```python
from build123d import *

# Parameters (mm, degrees)
SKETCH1_W           = 86.9
SKETCH1_H           = 86.9
BOSS_EXTRUDE1_DEPTH = 2
SKETCH2_R           = 1.65
CUT_EXTRUDE3_DEPTH  = 123.911431527
SKETCH3_R           = 1.5
CUT_EXTRUDE4_DEPTH  = 10
SKETCH4_R           = 1.5
CUT_EXTRUDE5_DEPTH  = 10
SKETCH5_W           = 3.5
SKETCH5_H           = 75
SKETCH5_W_2         = 75
SKETCH5_H_2         = 3.5
CUT_EXTRUDE6_DEPTH  = 123.911431527


with BuildPart() as part:
    # Sketch1 → Boss-Extrude1 (new body)
    with BuildSketch(Plane(origin=(0, 0, 0), x_dir=(0, 1, 0), z_dir=(0, 0, 1))):
        with Locations((43.45, 43.45)):
            Rectangle(SKETCH1_W, SKETCH1_H)
    extrude(amount=BOSS_EXTRUDE1_DEPTH)

    # Sketch2 → Cut-Extrude3 (cut, through all)
    with BuildSketch(Plane.XY.offset(2)):
        with Locations((-84.05, 2.85)):
            Circle(SKETCH2_R)
        with Locations((-2.85, 2.85)):
            Circle(SKETCH2_R)
        with Locations((-2.85, 84.05)):
            Circle(SKETCH2_R)
        with Locations((-84.05, 84.05)):
            Circle(SKETCH2_R)
    extrude(amount=-CUT_EXTRUDE3_DEPTH, mode=Mode.SUBTRACT)

    # Sketch3 → Cut-Extrude4 (cut)
    with BuildSketch(Plane.XY.offset(2)):
        with Locations((-79.2, 62.2)):
            Circle(SKETCH3_R)
        with Locations((-41.7, 62.2)):
            Circle(SKETCH3_R)
        with Locations((-41.7, 24.7)):
            Circle(SKETCH3_R)
        with Locations((-79.2, 24.7)):
            Circle(SKETCH3_R)
    extrude(amount=-CUT_EXTRUDE4_DEPTH, mode=Mode.SUBTRACT)

    # Sketch4 → Cut-Extrude5 (cut)
    with BuildSketch(Plane.XY.offset(2)):
        with Locations((-31.5, 66.7)):
            Circle(SKETCH4_R)
        with Locations((-8.5, 66.7)):
            Circle(SKETCH4_R)
        with Locations((-8.5, 20.2)):
            Circle(SKETCH4_R)
        with Locations((-31.5, 20.2)):
            Circle(SKETCH4_R)
    extrude(amount=-CUT_EXTRUDE5_DEPTH, mode=Mode.SUBTRACT)

    # Sketch5 → Cut-Extrude6 (cut, through all)
    with BuildSketch(Plane.XY.offset(2)):
        with Locations((-1.75, 43.45)):
            Rectangle(SKETCH5_W, SKETCH5_H)
        with Locations((-43.45, 85.15)):
            Rectangle(SKETCH5_W_2, SKETCH5_H_2)
    extrude(amount=-CUT_EXTRUDE6_DEPTH, mode=Mode.SUBTRACT)


solid = part.part
```
Here's how the part is built. I have some questions about the finished solid (model axes, mm). A direction names the side the tool comes from. Coordinates: 2 decimals unless noted, no trailing zeros. Order: outer loops, then holes, each group sorted by start corner. A loop starts at its lowest first (then second) coordinate and runs counter-clockwise, first axis right, second up.
Item 1: I'm going to push flat-ended pins straight in: pin 1 Ø6 at (x, y) = (-11, 16.5) entering from -Z; pin 2 Ø0.6 at (x, z) = (-39, 1.5) entering from +Y; pin 3 Ø1 at (y, z) = (29.5, 1.5) entering from +X. Where does each tip first touch, or does it pass through?
Response values:
pin 1: stops at z = 0
pin 2: stops at y = 83.4
pin 3: stops at x = -3.5
Item 2: I need wall thicknesses on probe 1 along Y at (x, z) = (-2.85, 1.05); probe 2 along X at (y, z) = (84.05, 0.5); probe 3 along Y at (x, z) = (-84.05, 0.9). Which ranges of each line are inside material? Lowest first, please.
Response values:
probe 1: y = 0 to 1.2, 4.5 to 5.95, 80.95 to 82.4, 85.7 to 86.9
probe 2: x = -86.9 to -85.7, -82.4 to -80.95, -5.95 to -4.5, -1.2 to 0
probe 3: y = 0 to 1.2, 4.5 to 82.4, 85.7 to 86.9
Item 3: Thinking about a two-plate mould opening in Y: for faces 1 (the face through (-40.27, 25.15, 1.01)), 2 (the face through (-84, 86.9, 1)), 3 (the face through (0, 3, 1)), which applies, pulls with the +Y half, pulls with the -Y half, needs draft (parallel to the pull), parting line crosses it, or undercut?
Response values:
face 1: undercut
face 2: pulls with the +Y half
face 3: needs draft
Item 4: If we section it at B-B, the plane x = -79.2: List the corners of the cut face in (y, z) for me, then the cut area to 3 significant figures.
Response values:
outline: (0, 0) - (23.2, 0) - (23.2, 2) - (0, 2) - close; (26.2, 0) - (60.7, 0) - (60.7, 2) - (26.2, 2) - close; (63.7, 0) - (83.4, 0) - (83.4, 2) - (63.7, 2) - close
area: 155 mm2
Item 5: Which directions (+Z, -Z, +X, -X, +Y, -Y) give clear straight access to the entire face, cutting with the end or side of a thin tool? Please do faces 4 (the face through (-3.5, 43, 1)), 5 (the face through (-5.95, 85, 1)), 6 (the face through (-3, 86.9, 1)).
Response values:
face 4: +Z, -Z, +X
face 5: +Z, -Z, +Y
face 6: +Z, -Z, +X, -X, +Y
Item 6: If we section it at C-C, the plane z = 1.4: Give the number of separate pieces and of enclosed holes in the cut face, then the cut area to 3 significant figures.
Response values:
separate pieces: 1
enclosed holes: 12
area: 6,940 mm2
Item 7: If we section it at A-A, the plane y = 2.85: List the corners of the cut face in (x, z) for me.
Response values:
outline: (-86.9, 0) - (-85.7, 0) - (-85.7, 2) - (-86.9, 2) - close; (-82.4, 0) - (-4.5, 0) - (-4.5, 2) - (-82.4, 2) - close; (-1.2, 0) - (0, 0) - (0, 2) - (-1.2, 2) - close
Item 8: If we section it at D-D, the plane x = -14: List the corners of the cut face in (y, z) for me, then the cut area to 3 significant figures.
Response values:
outline: (0, 0) - (83.4, 0) - (83.4, 2) - (0, 2) - close
area: 167 mm2
